from build123d import *

# Parameters (mm, degrees)
SKETCH1_W           = 18.288
SKETCH1_H           = 2.54
BOSS_EXTRUDE1_DEPTH = 8.509
SKETCH2_W           = 1.524
SKETCH2_H           = 1.524
CUT_EXTRUDE1_DEPTH  = 5.9944


with BuildPart() as part:
    # Sketch1 → Boss-Extrude1 (new body)
    with BuildSketch(Plane(origin=(0, 0, 0), x_dir=(1, 0, 0), z_dir=(0, 1, 0))):
        Rectangle(SKETCH1_W, SKETCH1_H)
    extrude(amount=BOSS_EXTRUDE1_DEPTH)

    # Sketch2 → Cut-Extrude1 (cut)
    with BuildSketch(Plane(origin=(0, 8.509, 0), x_dir=(1, 0, 0), z_dir=(0, 1, 0))):
        with Locations((2.54, 0)):
            Rectangle(SKETCH2_W, SKETCH2_H)
        Rectangle(SKETCH2_W, SKETCH2_H)
        with Locations((5.08, 0)):
            Rectangle(SKETCH2_W, SKETCH2_H)
        with Locations((7.62, 0)):
            Rectangle(SKETCH2_W, SKETCH2_H)
        with Locations((-2.54, 0)):
            Rectangle(SKETCH2_W, SKETCH2_H)
        with Locations((-5.08, 0)):
            Rectangle(SKETCH2_W, SKETCH2_H)
        with Locations((-7.62, 0)):
            Rectangle(SKETCH2_W, SKETCH2_H)
    extrude(amount=-CUT_EXTRUDE1_DEPTH, mode=Mode.SUBTRACT)


solid = part.part
Verification items for the finished model (mm, model axes). A direction names the side the tool comes from. Round coordinates to 2 decimals unless told otherwise and drop trailing zeros. Loops run counter-clockwise (first coordinate to the right, second up) from the corner with the lowest first, then second, coordinate; pieces in that order, holes last. Notation, with made-up numbers: (27, 7.5) - (83, 7.5) arc R29 ccw to (83, 27.5) - close; hole circle Ø7 at (24.5, -16). An arc over 180 degrees is marked (long way). Use one line per item in the form item = value.
1. Gauge pin test, flat end, axial feed: pin 1 Ø0.5 at (x, z) = (0, 0) entering from +Y. Record the tip position at first contact, or that the pin passes through.
A:
pin_1 = 2.51
2. Section check B-B on x = 7.25. Record the cut outline in (y, z), and give its area (3 significant figures).
A:
outline = (0, -1.27) - (8.51, -1.27) - (8.51, -0.76) - (2.51, -0.76) - (2.51, 0.76) - (8.51, 0.76) - (8.51, 1.27) - (0, 1.27) - close
area = 12.5 mm²
3. Draft check along Z on faces 3 (the flat face through (-5, 6, 0.762)), 4 (the flat face through (0.762, 6, 0)), 5 (the flat face through (0, 4, -1.27)), 6 (the flat face through (9.144, 4, 0)). Enter one of: pulls with the +Z half, pulls with the -Z half, needs draft (parallel to the pull), parting line crosses it, or undercut.
A:
face_3 = undercut
face_4 = undercut
face_5 = pulls with the -Z half
face_6 = needs draft
4. Scan lines: probe 1 along Z at (x, y) = (4.5, 2.75); probe 2 along Y at (x, z) = (-4.5, 0.45). Record each from-to range of solid material in increasing order.
A:
probe_1 = -1.27 to -0.76, 0.76 to 1.27
probe_2 = 0 to 2.51
5. Section check A-A on y = 5. Give the number of separate pieces and of enclosed holes in the cut face, and give its area (3 significant figures).
A:
separate_pieces = 1
enclosed_holes = 7
area = 30.2 mm²
6. Access from +Z, -Z, +X, -X, +Y, -Y to the whole of each face (thin tool, end or side, straight path). Record for faces 1 (the flat face through (0, 4, 1.27)), 2 (the flat face through (0, 6, 0.762)).
A:
face_1 = +Z, +X, -X, +Y, -Y
face_2 = +Y
